Autodesk Inventor part; units mm, degrees
ref_plane "YZ Plane" through (0, 0, 0) normal (1, 0, 0) x (0, 1, 0)
ref_plane "XZ Plane" through (0, 0, 0) normal (0, 1, 0) x (-1, 0, 0)
ref_plane "XY Plane" through (0, 0, 0) normal (0, 0, 1) x (1, 0, 0)
sketch "スケッチ1" plane through (0, 0, 0) normal (1, 0, 0) x (0, 1, 0)
  line L0 (-33.5119, 20.1143) -> (-33.5119, -204.2217)
  line L1 (6.4881, -204.2217) -> (6.4881, 20.1143)
  arc A0 (6.4881, 20.1143) -> (-33.5119, 20.1143) centre (-13.5119, 20.1143) ccw
  arc A1 (-33.5119, -204.2217) -> (6.4881, -204.2217) centre (-13.5119, -204.2217) ccw
  point P0 (0, 0)
  dimension "d2" = 224.336
  dimension "d3" = 224.336
  dimension "d4" = 40
  dimension "d5" = 40
extrude "押し出し1" add sketch "スケッチ1" along normal blind 40
sketch "スケッチ2" plane through (40, 0, 0) normal (1, 0, 0) x (0, 0, -1)
  line L0 (-19.9546, 4.6181) -> (204.3814, 4.6181)
  line L1 (204.3814, -31.6419) -> (-19.9546, -31.6419)
  line L2 (204.2217, 6.4881) -> (-20.1143, 6.4881)
  arc A0 (-19.9546, 4.6181) -> (-19.9546, -31.6419) centre (-19.9546, -13.5119) ccw
  arc A1 (204.3814, -31.6419) -> (204.3814, 4.6181) centre (204.3814, -13.5119) ccw
  point P0 (0, 0)
  dimension "d10" = 1.87
  dimension "d11" = 224.336
  dimension "d12" = 224.336
  dimension "d13" = 36.26
  dimension "d14" = 36.26
  dimension "d15" = 36.26
  dimension "d16" = 36.26
  dimension "d17" = 36.26
extrude "押し出し2" cut sketch "スケッチ2" against normal blind 40
properties part number "nhk11" material "ゴム"
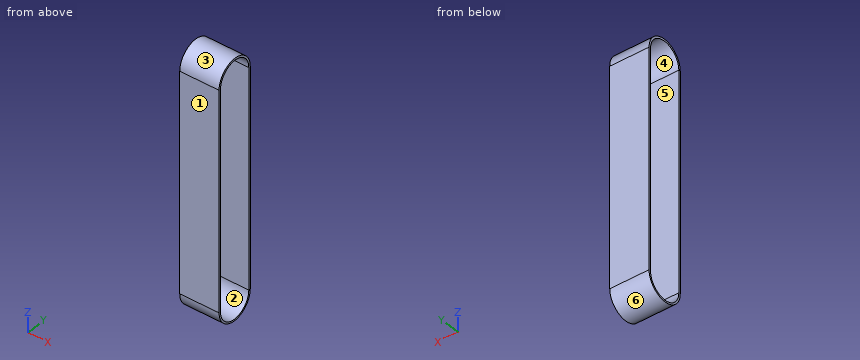
Work out the finished part from the listing and answer in its coordinate system (mm). Face numbers are marked on the shaded views. A direction names the side the tool comes from. Give positions to 0.01 mm unless a question says otherwise; leave off trailing zeros. Loops run counter-clockwise (first coordinate to the right, second up) from the corner with the lowest first, then second, coordinate; pieces in that order, holes last. Notation, with made-up numbers: (45.25, 32.25) -> (103.25, 32.25) arc R29 cw to (103.25, 53.25) -> close; hole circle Ø11 at (-19.75, 17.25). An arc over 180 degrees is marked (long way). Use a Markdown table: item, result. Add a question column.
1) Which of the six approach directions +Z, -Z, +X, -X, +Y, -Y give full straight-line access (tool end or side, diameter ignored) to the marked faces 1 and 2?
2) The part is cut by section C-C, the plane x = 5.5. Determine the outline of the cut face in (y, z), plus the area to 3 significant figures.
3) The part is cut by section B-B, the plane y = -14. Determine the outline of the cut face in (x, z).
4) For a pull along Z with two mould halves and no side action, classify the marked faces 3, 4, 5 and 6 as +Z half, -Z half, draft (parallel to the pull), parting line (faces both ways), or undercut.
5) The part is cut by section A-A, the plane z = -27.5. Determine the outline of the cut face in (x, y).
6) Each of these flat-tipped pins is pushed along its axis until it touches: P1, Ø4, axis at x = 28.5, y = -3, coming from the +Z side; P2, Ø4, axis at x = 16.5, y = -12.5, coming from the -Z side; P3, Ø5, axis at x = 17, y = 2, coming from the +Z side. Where does it stop, or does it pass through?
7) Consider line 1 along Y through (x, z) = (38.5, -24.5); line 2 along Z through (x, y) = (21, -13); line 3 along Z through (x, y) = (16, -27). Determine where each line is inside the solid, lowest interval first.
Reported:
| question | item | result |
|---|---|---|
| 1 | face 1 | +Z, -Z, +X, -X, -Y |
| 1 | face 2 | +X, -X |
| 2 | outline | (-33.51, -204.22) arc R20 ccw to (6.49, -204.22) -> (6.49, 20.11) arc R20 ccw to (-33.51, 20.11) -> close; hole (-31.64, -204.38) arc R18.13 ccw to (4.62, -204.38) -> (4.62, 19.95) arc R18.13 ccw to (-31.64, 19.95) -> close |
| 2 | area | 1,060 mm^2 |
| 3 | outline | (0, -224.22) -> (40, -224.22) -> (40, -222.5) -> (0, -222.5) -> close; (0, 38.08) -> (40, 38.08) -> (40, 40.11) -> (0, 40.11) -> close |
| 4 | face 3 | +Z half |
| 4 | face 4 | undercut |
| 4 | face 5 | undercut |
| 4 | face 6 | -Z half |
| 5 | outline | (0, -33.51) -> (40, -33.51) -> (40, -31.64) -> (0, -31.64) -> close; (0, 4.62) -> (40, 4.62) -> (40, 6.49) -> (0, 6.49) -> close |
| 6 | P1 | stops at z = 38.21 |
| 6 | P2 | stops at z = -224.22 |
| 6 | P3 | stops at z = 35.3 |
| 7 | line 1 | y = -33.51 to -31.64, 4.62 to 6.49 |
| 7 | line 2 | z = -224.22 to -222.5, 38.08 to 40.11 |
| 7 | line 3 | z = -218.99 to -216.5, 32.07 to 34.88 |
